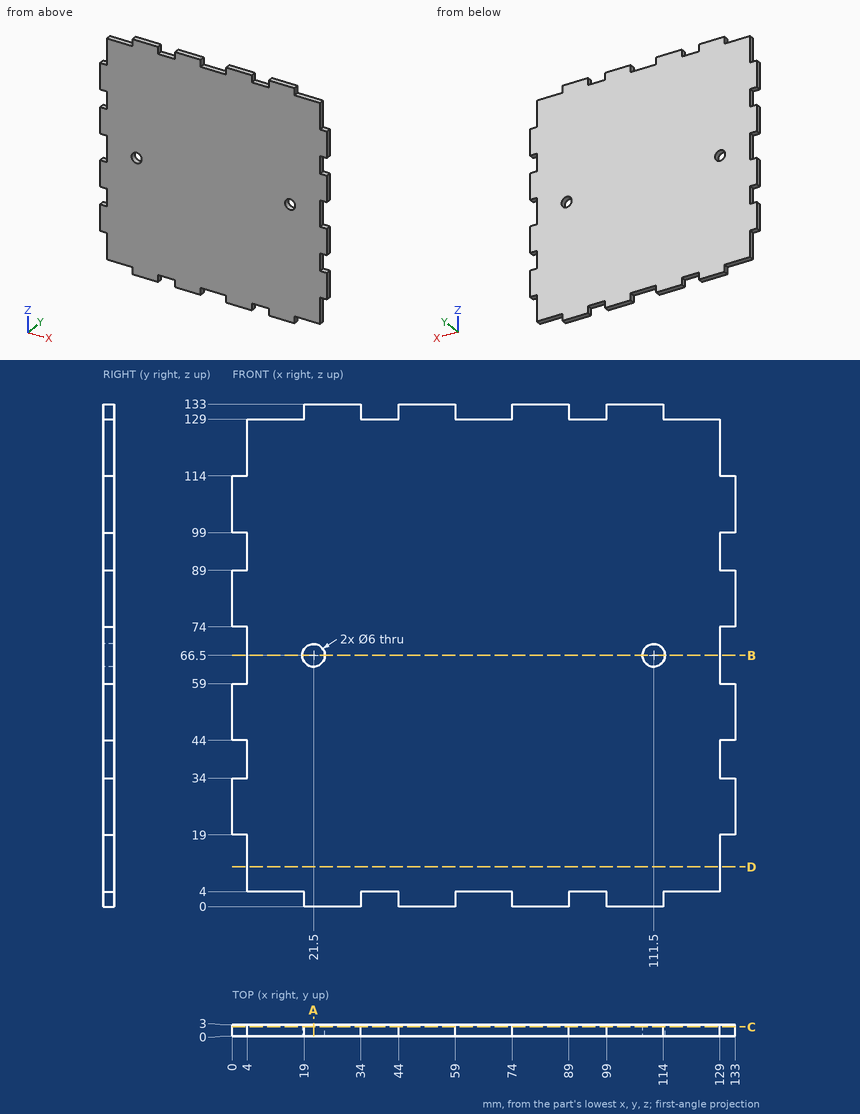
The figure shows three views and two pictorial views of one solid part (mm, origin at its lowest corner). Answer the questions. Coordinates: 2 decimals unless noted, no trailing zeros. Write each loop counter-clockwise with the first axis right and the second up, starting at its lowest first coordinate (ties: lowest second). Pieces come first, ordered by that corner, then holes. Notation, with made-up numbers: (-28.5, 12.25) -> (10.5, 12.25) arc R15 cw to (10.5, 23.25) -> close; hole circle Ø3 at (-16, 27.5). An arc over 180 degrees is marked (long way). Return JSON: item names as keys, results as strings.
1. A cutting plane is placed at C-C (y = 2.4). Give the number of separate pieces and of enclosed holes in the cut face, and give its area (3 significant figures).
Found:
{"separate pieces": "1", "enclosed holes": "2", "area": "16,500 mm2"}
2. Each of these flat-tipped pins is pushed along its axis until it touches: P1, Ø0.9, axis at x = 131.5, y = 2, coming from the +Z side; P2, Ø1.5, axis at x = 93, y = 2, coming from the -Z side; P3, Ø0.9, axis at x = 95.5, y = 1.5, coming from the +Z side. Where does it stop, or does it pass through?
Found:
{"P1": "z = 114", "P2": "z = 4", "P3": "z = 129"}
3. A cutting plane is placed at A-A (x = 21.5). Determine the outline of the cut face in (y, z).
Found:
{"outline": "(0, 0) -> (3, 0) -> (3, 63.5) -> (0, 63.5) -> close; (0, 69.5) -> (3, 69.5) -> (3, 133) -> (0, 133) -> close"}
4. A cutting plane is placed at D-D (z = 10.5). Determine the outline of the cut face in (x, y), and give its area (3 significant figures).
Found:
{"outline": "(4, 0) -> (129, 0) -> (129, 3) -> (4, 3) -> close", "area": "375 mm2"}
5. A cutting plane is placed at B-B (z = 66.5). Determine the outline of the cut face in (x, y).
Found:
{"outline": "(4, 0) -> (18.5, 0) -> (18.5, 3) -> (4, 3) -> close; (24.5, 0) -> (108.5, 0) -> (108.5, 3) -> (24.5, 3) -> close; (114.5, 0) -> (129, 0) -> (129, 3) -> (114.5, 3) -> close"}
6. Find the intervals of material crossed by line 1 along X through (y, z) = (1.75, 66.5); line 2 along Z through (x, y) = (21.5, 2); line 3 along X through (y, z) = (1.75, 117), in increasing order. Write a range as from..to.
Found:
{"line 1": "4..18.5, 24.5..108.5, 114.5..129", "line 2": "0..63.5, 69.5..133", "line 3": "4..129"}
